The figure shows three views and two pictorial views of one solid part (mm, origin at its lowest corner). Answer the questions. Give positions to 0.01 mm unless a question says otherwise; leave off trailing zeros. Order: outer loops, then holes, each group sorted by start corner. A loop starts at its lowest first (then second) coordinate and runs counter-clockwise, first axis right, second up. Notation, with made-up numbers: M -23.5,74 L 25.5,74 A27 cw 25.5,105 Z; hole C -20.75,33.5 d2. An arc over 180 degrees is marked long. One line per item, written item: value.
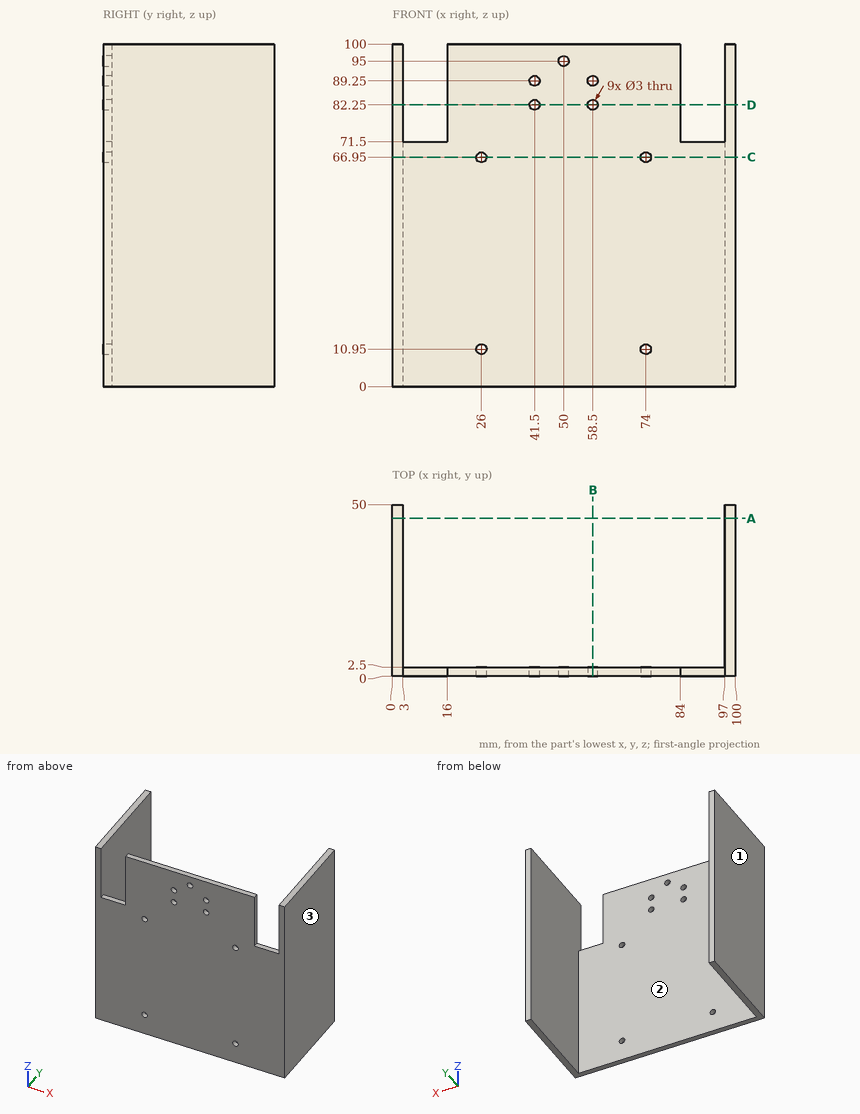
1) Determine the mould class of the marked faces 1, 2 and 3 for opening direction X: +X half, -X half, draft (parallel to the pull), parting line (faces both ways), or undercut.
Reported:
face 1: -X half
face 2: undercut
face 3: +X half
2) Find section B-B, the plane x = 58.5. Write down the section's boundary in (y, z), plus the area to 3 significant figures.
Reported:
outline: M 0,0 L 2.5,0 L 2.5,80.75 L 0,80.75 Z; M 0,83.75 L 2.5,83.75 L 2.5,87.75 L 0,87.75 Z; M 0,90.75 L 2.5,90.75 L 2.5,100 L 0,100 Z
area: 235 mm^2
3) Each of these flat-tipped pins is pushed along its axis until it touches: pin 1 Ø2 at (x, z) = (39.5, 70) entering from +Y; pin 2 Ø3 at (x, y) = (90.5, 1) entering from +Z. Where does it stop, or does it pass through?
Reported:
pin 1: stops at y = 2.5
pin 2: stops at z = 71.5
4) Consider probe 1 along X at (y, z) = (1.5, 82.25); probe 2 along X at (y, z) = (1, 95); probe 3 along Z at (x, y) = (74, 1). Determine where each line is inside the solid, lowest interval first.
Reported:
probe 1: x = 0 to 3, 16 to 40, 43 to 57, 60 to 84, 97 to 100
probe 2: x = 0 to 3, 16 to 48.5, 51.5 to 84, 97 to 100
probe 3: z = 0 to 9.45, 12.45 to 65.45, 68.45 to 100
5) Find section A-A, the plane y = 46. Write down the section's boundary in (x, z), plus the area to 3 significant figures.
Reported:
outline: M 0,0 L 3,0 L 3,100 L 0,100 Z; M 97,0 L 100,0 L 100,100 L 97,100 Z
area: 600 mm^2
6) Find section C-C, the plane z = 66.95. Write down the section's boundary in (x, y), plus the area to 3 significant figures.
Reported:
outline: M 0,0 L 24.5,0 L 24.5,2.5 L 3,2.5 L 3,50 L 0,50 Z; M 27.5,0 L 72.5,0 L 72.5,2.5 L 27.5,2.5 Z; M 75.5,0 L 100,0 L 100,50 L 97,50 L 97,2.5 L 75.5,2.5 Z
area: 520 mm^2
7) Find section D-D, the plane z = 82.25. Write down the section's boundary in (x, y), plus the area to 3 significant figures.
Reported:
outline: M 0,0 L 3,0 L 3,50 L 0,50 Z; M 16,0 L 40,0 L 40,2.5 L 16,2.5 Z; M 43,0 L 57,0 L 57,2.5 L 43,2.5 Z; M 60,0 L 84,0 L 84,2.5 L 60,2.5 Z; M 97,0 L 100,0 L 100,50 L 97,50 Z
area: 455 mm^2
